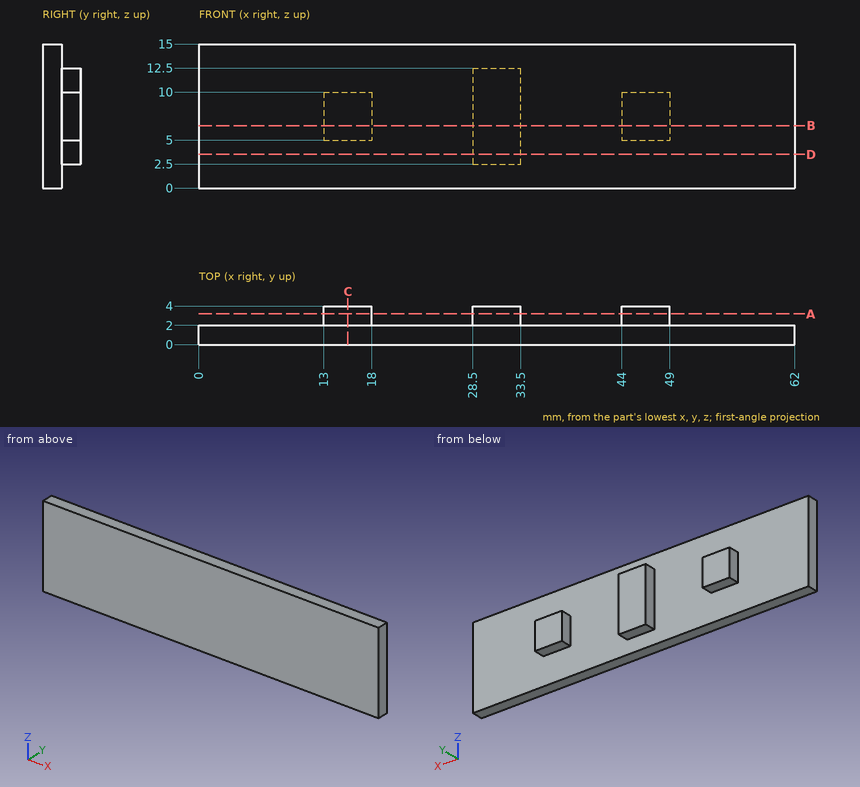
Part print with two shaded views. Sizes in mm from the minimum x, y, z corner. Round coordinates to 2 decimals unless told otherwise and drop trailing zeros. Order: outer loops, then holes, each group sorted by start corner. A loop starts at its lowest first (then second) coordinate and runs counter-clockwise, first axis right, second up. Notation, with made-up numbers: M 0,-26 L 21,-26 A25 cw 21,-4 Z; hole C 68,21.25 d11. An arc over 180 degrees is marked long. Answer in a Markdown table with one row per item. Add a question column.
Q1. Cut at D-D on z = 3.5. Give the cut face in (x, y).
Q2. Cut at A-A on y = 3.2. Give the cut face in (x, z), and give its area (3 significant figures).
Q3. Wall check: L1, parallel to X at y = 2.6, z = 9; L2, parallel to Y at x = 7.5, z = 4; L3, parallel to Z at x = 30.5, y = 3.55. Give the ranges that are in metal, low to high. Write a range as from..to.
Q4. Cut at B-B on z = 6.5. Give the cut face in (x, y).
Q5. Pin check, flat tips, straight feed: pin 1 (0.6 mm diameter, centred on x = 46.5, y = 3.5, fed in from -Z); pin 2 (1 mm diameter, centred on y = 3.5, z = 8.5, fed in from +X); pin 3 (4 mm diameter, centred on x = 9, z = 7, fed in from +Y). Stop position of each tip, or through.
Q6. Cut at C-C on x = 15.5. Give the cut face in (y, z).
Established:
| question | item | result |
|---|---|---|
| 1 | outline | M 0,0 L 62,0 L 62,2 L 33.5,2 L 33.5,4 L 28.5,4 L 28.5,2 L 0,2 Z |
| 2 | outline | M 13,5 L 18,5 L 18,10 L 13,10 Z; M 28.5,2.5 L 33.5,2.5 L 33.5,12.5 L 28.5,12.5 Z; M 44,5 L 49,5 L 49,10 L 44,10 Z |
| 2 | area | 100 mm2 |
| 3 | L1 | x = 13..18, 28.5..33.5, 44..49 |
| 3 | L2 | y = 0..2 |
| 3 | L3 | z = 2.5..12.5 |
| 4 | outline | M 0,0 L 62,0 L 62,2 L 49,2 L 49,4 L 44,4 L 44,2 L 33.5,2 L 33.5,4 L 28.5,4 L 28.5,2 L 18,2 L 18,4 L 13,4 L 13,2 L 0,2 Z |
| 5 | pin 1 | stops at z = 5 |
| 5 | pin 2 | stops at x = 49 |
| 5 | pin 3 | stops at y = 2 |
| 6 | outline | M 0,0 L 2,0 L 2,5 L 4,5 L 4,10 L 2,10 L 2,15 L 0,15 Z |
